```python
from build123d import *


with BuildPart() as part:
    # Sketch1 → Revolve1 (revolve)
    with BuildSketch(Plane(origin=(0, 0, 0), x_dir=(1, 0, 0), z_dir=(0, 1, 0))):
        with BuildLine():
            Line((0, 0), (0, -108.493072777))
            Line((0, -108.493072777), (1.647963045, -108.493072777))
            add(Edge.make_bspline(
                [(6.504116771, -37.330573794), (5.545242456, -73.016533956), (1.647963045, -108.493072777)],
                knots=[0, 0, 0, 1, 1, 1], degree=2))
            Line((6.504116771, -37.330573794), (5.508233542, -36.334690565))
            Line((5.508233542, -36.334690565), (5.508233542, -16.28474128))
            Line((5.508233542, -16.28474128), (7.5, -14.292974822))
            Line((7.5, -14.292974822), (7.5, 0))
            Line((7.5, 0), (0, 0))
        make_face()
    revolve(axis=Axis((0, 0, 0), (0, 0, 1)))


solid = part.part
```
Geometry check sheet. Reference: the model listing, model coordinates, mm. Give positions to 0.01 mm unless a question says otherwise; leave off trailing zeros. Write each loop counter-clockwise with the first axis right and the second up, starting at its lowest first coordinate (ties: lowest second). Pieces come first, ordered by that corner, then holes.
1) Section check A-A, the plane z = 29. Record the boundary of the cut face in (x, y).
2) Material ranges on L1, parallel to X at y = 0.75, z = 100; L2, parallel to X at y = 3.75, z = 33; L3, parallel to Y at x = 1.75, z = 18, recorded low to high.
3) Gauge pin test, flat ends, axial feed: pin 1 (2 mm diameter, centred on y = -2.5, z = 35.5, fed in from -X); pin 2 (4 mm diameter, centred on y = 2, z = 24, fed in from -X); pin 3 (4 mm diameter, centred on x = 3, y = 5.5, fed in from -Z); pin 4 (5 mm diameter, centred on y = -4.5, z = 60, fed in from +X). Record the tip position at first contact, or that the pin passes through.
4) Release check for a two-part mould opening along Z. For faces 1 (the flat face through (0, 0, 0)), 2 (the flat face through (0, 0, 108.493)), 3 (the cylindrical face through (-7.493, 0.33, 7.046)), 4 (the conical face through (-1.22, -5.5, 16.16)) record: pulls with the +Z half, pulls with the -Z half, needs draft (parallel to the pull), parting line crosses it, or undercut.
Computed:
1. outline: circle Ø11.02 at (0, 0)
2. L1: x = -2.43 to 2.43
2. L2: x = -4.03 to 4.03
2. L3: y = -5.22 to 5.22
3. pin 1: stops at x = -5.3
3. pin 2: stops at x = -5.51
3. pin 3: stops at z = 0
3. pin 4: stops at x = 5.24
4. face 1: pulls with the -Z half
4. face 2: pulls with the +Z half
4. face 3: needs draft
4. face 4: undercut
